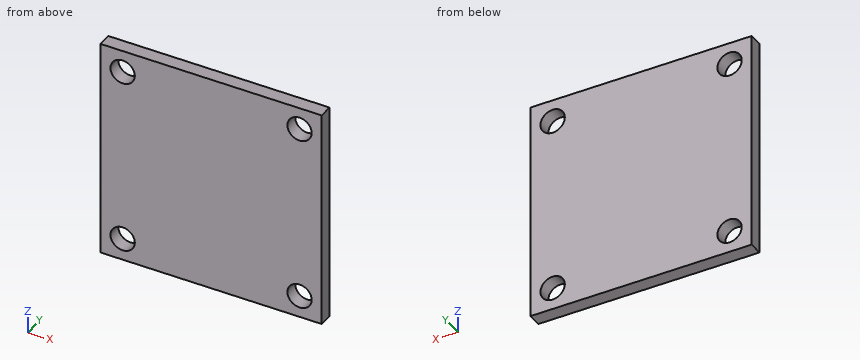
```python
from build123d import *

# Parameters (mm, degrees)
ESBO_O1_W                 = 200
ESBO_O1_H                 = 200
RESSALTO_EXTRUS_O1_DEPTH  = 12.5
ESBO_O2_R                 = 11
CORTE_EXTRUS_O1_DEPTH     = 142.972708645
PADR_O_LINEAR1_COUNT      = 2
PADR_O_LINEAR1_PITCH      = 160
PADR_O_LINEAR1_COUNT_DIR2 = 2
PADR_O_LINEAR1_PITCH_DIR2 = 160


with BuildPart() as part:
    # Esboço1 → Ressalto-extrusão1 (new body)
    with BuildSketch(Plane(origin=(0, 0, 0), x_dir=(1, 0, 0), z_dir=(0, 1, 0))):
        Rectangle(ESBO_O1_W, ESBO_O1_H)
    extrude(amount=RESSALTO_EXTRUS_O1_DEPTH)

    # Esboço2 → Corte-extrusão1 (cut, through all)
    with BuildSketch(Plane(origin=(0, 12.5, 0), x_dir=(1, 0, 0), z_dir=(0, 1, 0))):
        with Locations(Location((-80, 80, 0), (0, 0, 270))):
            Circle(ESBO_O2_R)
    corte_extrus_o1 = extrude(amount=-CORTE_EXTRUS_O1_DEPTH, mode=Mode.SUBTRACT)

    # Padrão linear1: Corte-extrus_o1 2 × 2
    with Locations(*[(i * PADR_O_LINEAR1_PITCH, 0, j * PADR_O_LINEAR1_PITCH_DIR2) for i in range(PADR_O_LINEAR1_COUNT) for j in range(PADR_O_LINEAR1_COUNT_DIR2) if (i, j) != (0, 0)]):
        add(corte_extrus_o1, mode=Mode.SUBTRACT)


solid = part.part
```
Can you work these out from the model? Positions are in its coordinate system, mm. Coordinates: 2 decimals unless noted, no trailing zeros. Order: outer loops, then holes, each group sorted by start corner. A loop starts at its lowest first (then second) coordinate and runs counter-clockwise, first axis right, second up.
1. If we section it at C-C (x = 80): Please give me the cut outline in (y, z).
2. I'm going to push a flat-ended pin straight in: pin 1 (20 mm diameter, centred on x = 80, z = -80, fed in from +Y). Where does the tip first touch, or does it pass through?
3. I need wall thicknesses on line 1 (X direction, y = 4.5, z = -80); line 2 (Z direction, x = -83.5, y = 3.5); line 3 (X direction, y = 10.75, z = 74.5). Which ranges of each line are inside material? Lowest first, please.
4. If we section it at B-B (y = 10): Please give me the cut outline in (x, z), then the cut area to 3 significant figures.
5. If we section it at A-A (z = -80): Please give me the cut outline in (x, y).
Entries:
1. outline: (0, -100) - (12.5, -100) - (12.5, -91) - (0, -91) - close; (0, -69) - (12.5, -69) - (12.5, 69) - (0, 69) - close; (0, 91) - (12.5, 91) - (12.5, 100) - (0, 100) - close
2. pin 1: passes through
3. line 1: x = -100 to -91, -69 to 69, 91 to 100
3. line 2: z = -100 to -90.43, -69.57 to 69.57, 90.43 to 100
3. line 3: x = -100 to -89.53, -70.47 to 70.47, 89.53 to 100
4. outline: (-100, -100) - (100, -100) - (100, 100) - (-100, 100) - close; hole circle Ø22 at (-80, -80); hole circle Ø22 at (-80, 80); hole circle Ø22 at (80, -80); hole circle Ø22 at (80, 80)
4. area: 38,500 mm2
5. outline: (-100, 0) - (-91, 0) - (-91, 12.5) - (-100, 12.5) - close; (-69, 0) - (69, 0) - (69, 12.5) - (-69, 12.5) - close; (91, 0) - (100, 0) - (100, 12.5) - (91, 12.5) - close
